Geometry: final body of the model. Coordinates: model frame, mm. Face numbers are marked on the shaded views. A direction names the side the tool comes from. Coordinates: 2 decimals unless noted, no trailing zeros. One line per item, written item: value. Start each with the question number.
from build123d import *

# Parameters (mm, degrees)
SKETCH1_W           = 151
SKETCH1_H           = 65
BOSS_EXTRUDE1_DEPTH = 94
SKETCH2_W           = 151
SKETCH2_H           = 65
SKETCH2_W_2         = 149
SKETCH2_H_2         = 63
CUT_EXTRUDE1_DEPTH  = 15
SKETCH3_W           = 130
SKETCH3_H           = 1
CUT_EXTRUDE2_DEPTH  = 7.5
SKETCH4_W           = 1
SKETCH4_H           = 35
CUT_EXTRUDE3_DEPTH  = 7.5


with BuildPart() as part:
    # Sketch1 → Boss-Extrude1 (new body)
    with BuildSketch(Plane(origin=(0, 0, 0), x_dir=(1, 0, 0), z_dir=(0, 1, 0))):
        Rectangle(SKETCH1_W, SKETCH1_H)
    extrude(amount=BOSS_EXTRUDE1_DEPTH)

    # Sketch2 → Cut-Extrude1 (cut)
    with BuildSketch(Plane(origin=(0, 94, 0), x_dir=(1, 0, 0), z_dir=(0, 1, 0))):
        Rectangle(SKETCH2_W, SKETCH2_H)
        Rectangle(SKETCH2_W_2, SKETCH2_H_2, mode=Mode.SUBTRACT)
    extrude(amount=-CUT_EXTRUDE1_DEPTH, mode=Mode.SUBTRACT)

    # Sketch3 → Cut-Extrude2 (cut)
    with BuildSketch(Plane(origin=(0, 94, 0), x_dir=(1, 0, 0), z_dir=(0, 1, 0))):
        with Locations((9.5, 31)):
            Rectangle(SKETCH3_W, SKETCH3_H)
        with Locations((9.5, -31)):
            Rectangle(SKETCH3_W, SKETCH3_H)
    extrude(amount=-CUT_EXTRUDE2_DEPTH, mode=Mode.SUBTRACT)

    # Sketch4 → Cut-Extrude3 (cut)
    with BuildSketch(Plane(origin=(0, 94, 0), x_dir=(1, 0, 0), z_dir=(0, 1, 0))):
        with Locations((-74, 0)):
            Rectangle(SKETCH4_W, SKETCH4_H)
    extrude(amount=-CUT_EXTRUDE3_DEPTH, mode=Mode.SUBTRACT)


solid = part.part
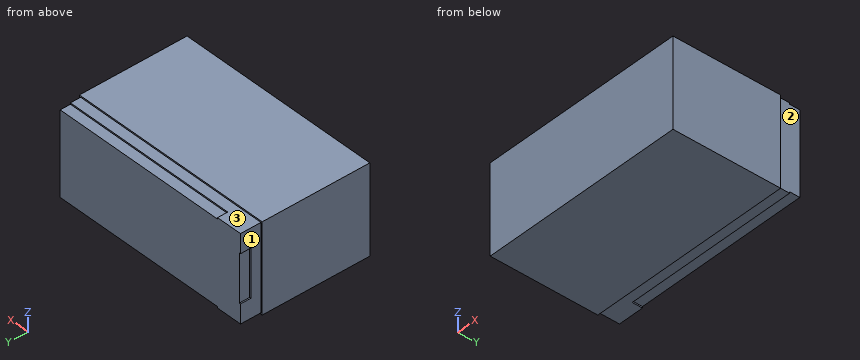
Q1. Access query for the marked faces 1, 2 and 3. Directions: +Z, -Z, +X, -X, +Y, -Y. A direction counts if a zero-diameter tool reaches every point of the face in a straight line with its end or side. Return the directions, or none.
Q2. First-contact query: P1, Ø0.8, axis at x = -74, y = 88.5, coming from the -Z side; P2, Ø6, axis at x = 37, y = 89, coming from the +Z side; P3, Ø2, axis at x = -49, z = -3, coming from the -Y side; P4, Ø4.5, axis at y = 84.5, z = -8.5, coming from the +X side. Flat tips, straight axial feed; report the tip coordinate or a pass-through.
Q3. Line query: L1, parallel to X at y = 87, z = 26; L2, parallel to Z at x = 47.5, y = 82; L3, parallel to X at y = 89.5, z = -16.5. Output: solid intervals per line, ascending. Write a range as from..to.
Solution:
1. face 1: +Z, -Z, -X, +Y
1. face 2: +Z, -Z, +X, +Y
1. face 3: +Z, +X, -X, +Y
2. P1: z = -31.5
2. P2: z = 31.5
2. P3: y = 0
2. P4: x = 74.5
3. L1: -74.5..74.5
3. L2: -31.5..31.5
3. L3: -73.5..74.5
